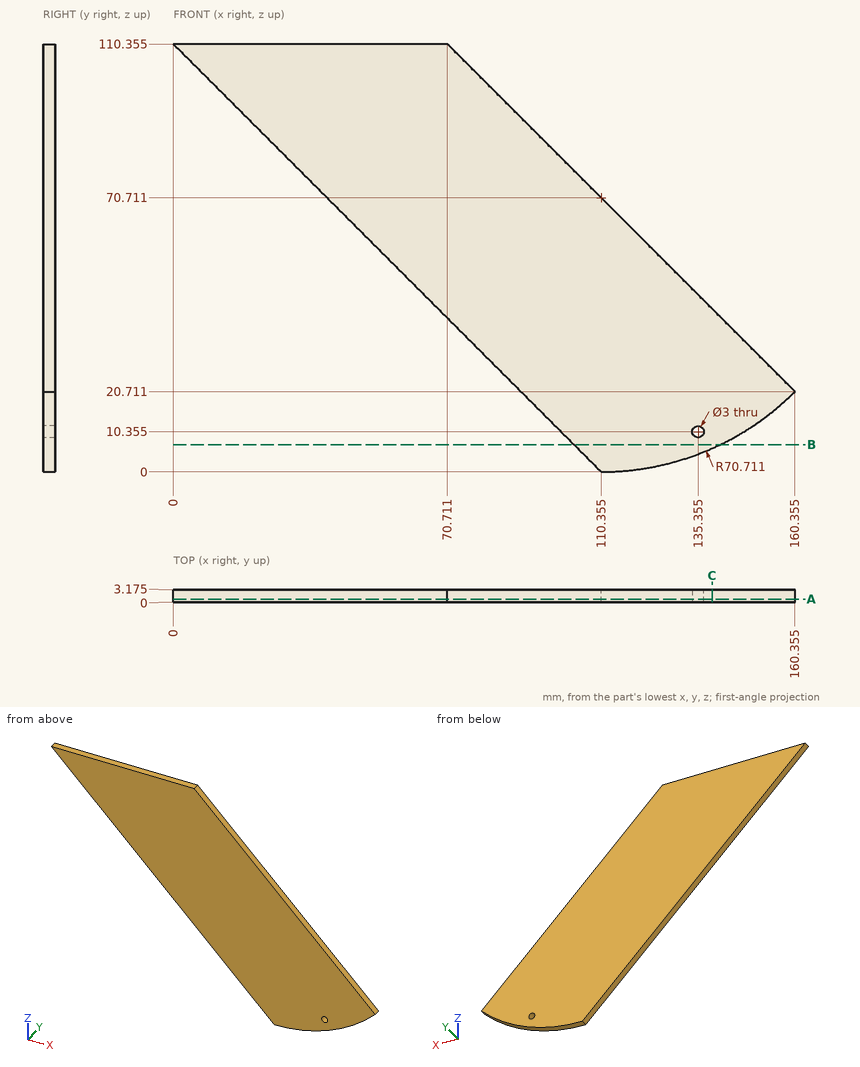
Study the drawing (mm; zero at the part's minimum x, y, z) and answer. Give positions to 0.01 mm unless a question says otherwise; leave off trailing zeros. Order: outer loops, then holes, each group sorted by start corner. A loop starts at its lowest first (then second) coordinate and runs counter-clockwise, first axis right, second up.
1) Find section B-B on z = 7. Write down the section's boundary in (x, y) (1 decimal).
Reported:
outline: (103.4, 0) - (141, 0) - (141, 3.2) - (103.4, 3.2) - close
2) Given P1, Ø2.5, axis at x = 135.36, z = 10.36, coming from the -Y side; P2, Ø1.5, axis at y = 0.5, z = 17, coming from the +X side; P3, Ø1, axis at y = 2, z = 20, coming from the +X side (1 decimal), each flat-ended and moving along its own axis, determine where each tip first touches the part or whether it passes through.
Reported:
P1: passes through
P2: stops at x = 157.21
P3: stops at x = 160.1
3) Consider line 1 along Z through (x, y) = (136, 0.9) (1 decimal); line 2 along Z through (x, y) = (60, 0.5) (1 decimal); line 3 along Z through (x, y) = (8, 2.9) (1 decimal). Determine where each line is inside the solid, lowest interval first.
Reported:
line 1: z = 4.8 to 9, 11.7 to 45.1
line 2: z = 50.4 to 110.4
line 3: z = 102.4 to 110.4
4) Find section A-A on y = 0.8. Write down the section's boundary in (x, z) (1 decimal), then the cut area to 3 significant figures.
Reported:
outline: (0, 110.4) - (110.4, 0) arc R70.7 ccw to (160.4, 20.7) - (70.7, 110.4) - close; hole circle Ø3 at (135.4, 10.4)
area: 7,260 mm2
5) Find section C-C on x = 139. Write down the section's boundary in (y, z) (1 decimal).
Reported:
outline: (0, 6.1) - (3.2, 6.1) - (3.2, 42.1) - (0, 42.1) - close
